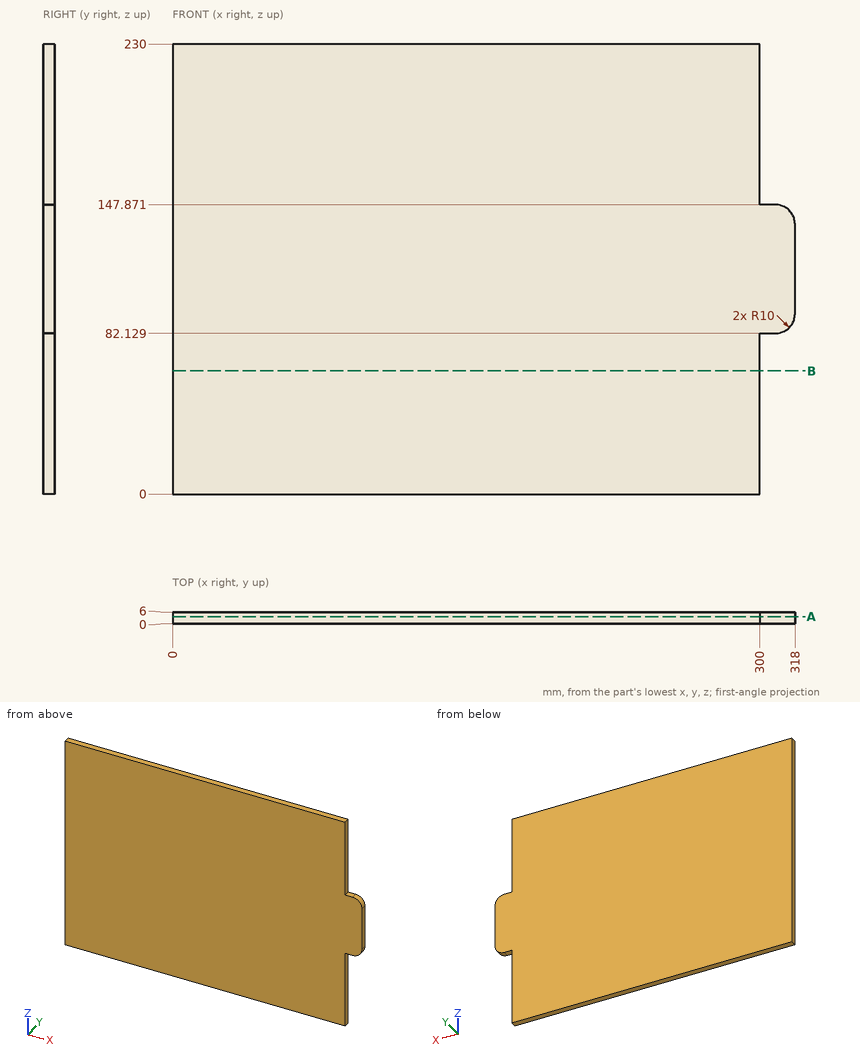
Source: three-view drawing plus pictorial views. Frame: mm from the lowest corner of the part. Give positions to 0.01 mm unless a question says otherwise; leave off trailing zeros. Loops run counter-clockwise (first coordinate to the right, second up) from the corner with the lowest first, then second, coordinate; pieces in that order, holes last. Notation, with made-up numbers: M -28.75,17.25 L -9.75,17.25 A22 cw -9.75,37.25 Z; hole C 89,27.25 d4. An arc over 180 degrees is marked long. Put each result on its own line as item: value.
Q1. Section A-A (y = 3.7). Return the cut outline in (x, z).
Response values:
outline: M 0,0 L 300,0 L 300,82.13 L 308,82.13 A10 ccw 318,92.13 L 318,137.87 A10 ccw 308,147.87 L 300,147.87 L 300,230 L 0,230 Z
Q2. Pin query (flat end, axial travel): P1, Ø1.8, axis at y = 3.5, z = 194.5, coming from the +X side; P2, Ø3, axis at x = 304.5, y = 2.5, coming from the -Z side. Return the tip coordinate at first contact, or that it passes through.
Response values:
P1: stops at x = 300
P2: stops at z = 82.13
Q3. Section B-B (z = 63). Return the cut outline in (x, y), and give its area (3 significant figures).
Response values:
outline: M 0,0 L 300,0 L 300,6 L 0,6 Z
area: 1,800 mm²
Q4. Line query: probe 1 along X at (y, z) = (4.3, 70); probe 2 along X at (y, z) = (0.75, 143.5). Output: solid intervals per line, ascending. Write a range as [from, to].
Response values:
probe 1: x = [0, 300]
probe 2: x = [0, 316.27]
